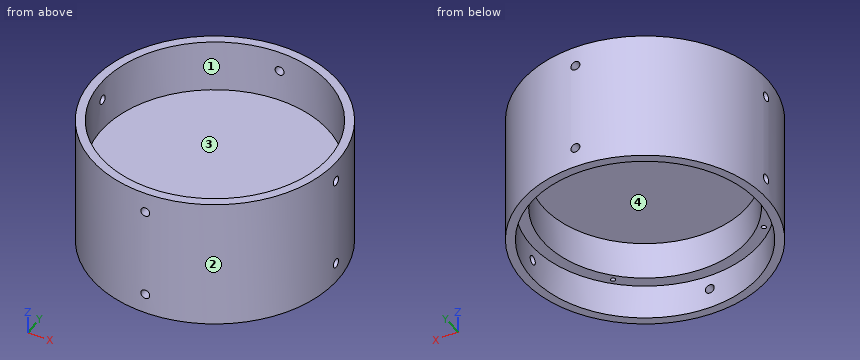
```python
from build123d import *

# Parameters (mm, degrees)
ESQUISSE1_R                  = 42
BOSS_EXTRU_1_DEPTH           = 33
R_P_TITION_CIRCULAIRE1_COUNT = 4
ESQUISSE5_R                  = 35
ENL_V_MAT_EXTRU_1_DEPTH      = 13
ESQUISSE7_R                  = 39
ENL_V_MAT_EXTRU_2_DEPTH      = 18
R_P_TITION_CIRCULAIRE2_COUNT = 4
ESQUISSE14_W                 = 3
ESQUISSE14_H                 = 12
R_P_TITION_CIRCULAIRE3_COUNT = 4


with BuildPart() as part:
    # Esquisse1 → Boss.-Extru.1 (new body)
    with BuildSketch(Plane.XY):
        Circle(ESQUISSE1_R)
    extrude(amount=BOSS_EXTRU_1_DEPTH)

    # Esquisse3 → Trou taraudé M21 (revolve, cut)
    with BuildSketch(Plane(origin=(-26.162950904, 26.162950904, 0), x_dir=(0, 1, 0), z_dir=(1, 0, 0))):
        Polygon((0, 0), (0, 6.480688495), (0.8, 6), (0.8, 0), align=None)
    trou_taraud_m21 = revolve(axis=Axis((-26.162950904, 26.162950904, -6.35), (0, 0, 1)), mode=Mode.SUBTRACT)

    # Répétition circulaire1: Trou taraudé M21 ×4 about axis
    r_p_tition_circulaire1_axis = Axis((0, 0, 0), (0, 0, 1))
    for i in range(1, R_P_TITION_CIRCULAIRE1_COUNT):
        add(trou_taraud_m21.rotate(r_p_tition_circulaire1_axis, i * 360 / R_P_TITION_CIRCULAIRE1_COUNT), mode=Mode.SUBTRACT)

    # Esquisse5 → Enlèv. mat.-Extru.1 (cut)
    with BuildSketch(Plane(origin=(0, 0, 0), x_dir=(-1, 0, 0), z_dir=(0, 0, -1))):
        Circle(ESQUISSE5_R)
    extrude(amount=-ENL_V_MAT_EXTRU_1_DEPTH, mode=Mode.SUBTRACT)

    # Esquisse7 → Enlèv. mat.-Extru.2 (cut)
    with BuildSketch(Plane.XY.offset(33)):
        Circle(ESQUISSE7_R)
    extrude(amount=-ENL_V_MAT_EXTRU_2_DEPTH, mode=Mode.SUBTRACT)

    # Esquisse13 → Dégagement M2.51 (revolve, cut)
    with BuildSketch(Plane(origin=(42, 0, 26), x_dir=(0, 0, -1), z_dir=(0, 1, 0))):
        Polygon((0, 0), (0, 10.931333959), (1.55, 10), (1.55, 0), align=None)
    d_gagement_m2_51 = revolve(axis=Axis((48.35, 0, 26), (-1, 0, 0)), mode=Mode.SUBTRACT)

    # Répétition circulaire2: Dégagement M2.51 ×4 about axis
    r_p_tition_circulaire2_axis = Axis((0, 0, 33), (0, 0, 1))
    for i in range(1, R_P_TITION_CIRCULAIRE2_COUNT):
        add(d_gagement_m2_51.rotate(r_p_tition_circulaire2_axis, i * 360 / R_P_TITION_CIRCULAIRE2_COUNT), mode=Mode.SUBTRACT)

    # Esquisse14 → Révolution1 (revolve)
    with BuildSketch(Plane(origin=(0, 0, 0), x_dir=(1, 0, 0), z_dir=(0, 1, 0))):
        with Locations((40.5, 6)):
            Rectangle(ESQUISSE14_W, ESQUISSE14_H)
    revolve(axis=Axis((0, 0, -20.123212499), (0, 0, 1)))

    # Esquisse15 → Dégagement M2.52 (revolve, cut)
    with BuildSketch(Plane(origin=(42, 0, -5), x_dir=(0, 0, -1), z_dir=(0, 1, 0))):
        Polygon((0, 0), (0, 9.431333959), (1.55, 8.5), (1.55, 0), align=None)
    d_gagement_m2_52 = revolve(axis=Axis((48.35, 0, -5), (-1, 0, 0)), mode=Mode.SUBTRACT)

    # Répétition circulaire3: Dégagement M2.52 ×4 about axis
    r_p_tition_circulaire3_axis = Axis((0, 0, 0), (0, 0, -1))
    for i in range(1, R_P_TITION_CIRCULAIRE3_COUNT):
        add(d_gagement_m2_52.rotate(r_p_tition_circulaire3_axis, i * 360 / R_P_TITION_CIRCULAIRE3_COUNT), mode=Mode.SUBTRACT)


solid = part.part
```
Can you work these out from the model? Positions are in its coordinate system, mm. Face numbers are marked on the shaded views. A direction names the side the tool comes from. Coordinates: 2 decimals unless noted, no trailing zeros. Order: outer loops, then holes, each group sorted by start corner. A loop starts at its lowest first (then second) coordinate and runs counter-clockwise, first axis right, second up.
1. If we section it at D-D (y = 12): Please give me the cut outline in (x, z).
2. If we section it at A-A (y = 0): Give the number of separate pieces and of enclosed holes in the cut face, then the cut area to 3 significant figures.
3. I'm going to push flat-ended pins straight in: pin 1 (10 mm diameter, centred on y = -32, z = -2.5, fed in from -X); pin 2 (6 mm diameter, centred on y = -15.5, z = 14.5, fed in from -X); pin 3 (2.5 mm diameter, centred on x = -26.16, y = 26.16, fed in from -Z). Where does each tip first touch, or does it pass through?
4. I need wall thicknesses on line 1 (Y direction, x = 0, z = 23); line 2 (Z direction, x = -13, y = -3); line 3 (Y direction, x = 21.5, z = 30). Which ranges of each line are inside material? Lowest first, please.
5. Thinking about a two-plate mould opening in X: for the marked faces 1 and 2, which applies, +X half, -X half, draft (parallel to the pull), parting line (faces both ways), or undercut?
6. For the marked faces 3 and 4, which set-ups out of +Z, -Z, +X, -X, +Y, -Y let a thin tool reach every point of the face, with its end or its side?
7. If we section it at C-C (z = -5): Please give me the cut outline in (x, y), then the cut area to 3 significant figures.
Entries:
1. outline: (-40.25, -12) - (-37.11, -12) - (-37.11, 0) - (-32.88, 0) - (-32.88, 13) - (32.88, 13) - (32.88, 0) - (37.11, 0) - (37.11, -12) - (40.25, -12) - (40.25, 33) - (37.11, 33) - (37.11, 15) - (-37.11, 15) - (-37.11, 33) - (-40.25, 33) - close
2. separate pieces: 5
2. enclosed holes: 0
2. area: 493 mm2
3. pin 1: stops at x = -32.17
3. pin 2: stops at x = -40.1
3. pin 3: stops at z = 0
4. line 1: y = -42 to -39, 39 to 42
4. line 2: z = 13 to 15
4. line 3: y = -36.08 to -32.54, 32.54 to 36.08
5. face 1: undercut
5. face 2: parting line
6. face 3: +Z
6. face 4: -Z
7. outline: (-41.97, -1.55) arc R42 ccw to (-1.55, -41.97) - (-1.55, -38.97) arc R39 cw to (-38.97, -1.55) - close; (-41.97, 1.55) - (-38.97, 1.55) arc R39 cw to (-1.55, 38.97) - (-1.55, 41.97) arc R42 ccw to start; (1.55, -41.97) arc R42 ccw to (41.97, -1.55) - (38.97, -1.55) arc R39 cw to (1.55, -38.97) - close; (1.55, 38.97) arc R39 cw to (38.97, 1.55) - (41.97, 1.55) arc R42 ccw to (1.55, 41.97) - close
7. area: 726 mm2
